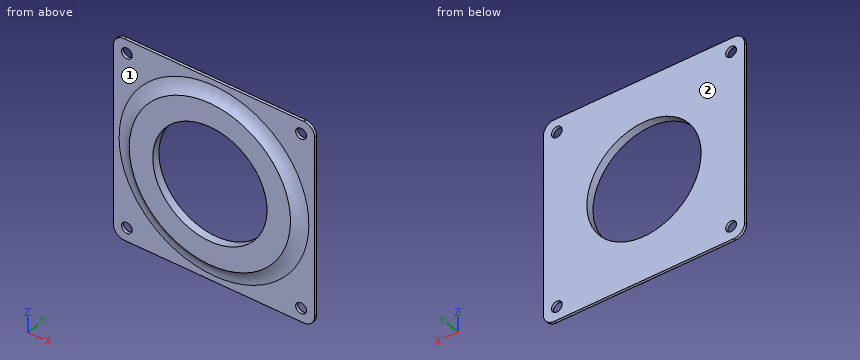
from build123d import *

# Parameters (mm, degrees)
BOSS_EXTRUDE1_DEPTH = 1.27
SKETCH2_R           = 38.1
BOSS_EXTRUDE2_DEPTH = 2.54
FILLET1_R           = 10.16
SKETCH3_R           = 27
CUT_EXTRUDE1_DEPTH  = 68.28310412
SKETCH4_R           = 2.54
CUT_EXTRUDE2_DEPTH  = 68.28310412


with BuildPart() as part:
    # Sketch1 → Boss-Extrude1 (new body)
    with BuildSketch(Plane(origin=(0, 0, 0), x_dir=(1, 0, 0), z_dir=(0, 1, 0))):
        with BuildLine():
            Line((-42.42, -47.5), (42.42, -47.5))
            ThreePointArc((42.42, -47.5), (46.012102448, -46.012102448), (47.5, -42.42))
            Line((47.5, -42.42), (47.5, 42.42))
            ThreePointArc((47.5, 42.42), (46.012102448, 46.012102448), (42.42, 47.5))
            Line((42.42, 47.5), (-42.42, 47.5))
            ThreePointArc((-42.42, 47.5), (-46.012102448, 46.012102448), (-47.5, 42.42))
            Line((-47.5, 42.42), (-47.5, -42.42))
            ThreePointArc((-47.5, -42.42), (-46.012102448, -46.012102448), (-42.42, -47.5))
        make_face()
    extrude(amount=BOSS_EXTRUDE1_DEPTH)

    # Sketch2 → Boss-Extrude2 (add)
    with BuildSketch(Plane.XZ):
        with Locations(Location((0, 0, 0), (0, 0, 270))):
            Circle(SKETCH2_R)
    extrude(amount=BOSS_EXTRUDE2_DEPTH)

    # Fillet1
    # the kernel refuses this fillet: 10.16 mm, written as the material it adds along each edge
    with BuildSketch(Plane(origin=(0, 0, 0), x_dir=(0, 0, -1), z_dir=(-1, 0, 0))) as fillet1_piece_1:
        with BuildLine():
            CenterArc((44.82020833, 10.16), FILLET1_R, 228.590377891, 41.409622109)
            Line((38.1, 2.54), (38.1, 0))
            Line((38.1, 0), (44.82020833, 0))
        make_face()
    revolve(axis=Axis((0, 0, 0), (0, -1, 0)))

    # Sketch3 → Cut-Extrude1 (cut, through all)
    with BuildSketch(Plane(origin=(0, 1.27, 0), x_dir=(1, 0, 0), z_dir=(0, 1, 0))):
        with Locations(Location((0, 0, 0), (0, 0, 270))):
            Circle(SKETCH3_R)
    extrude(amount=-CUT_EXTRUDE1_DEPTH, mode=Mode.SUBTRACT)

    # Sketch4 → Cut-Extrude2 (cut, through all)
    with BuildSketch(Plane(origin=(0, 1.27, 0), x_dir=(1, 0, 0), z_dir=(0, 1, 0))):
        with Locations(Location((-41.15, 41.15, 0), (0, 0, 270))):
            Circle(SKETCH4_R)
        with Locations(Location((41.15, 41.15, 0), (0, 0, 90))):
            Circle(SKETCH4_R)
        with Locations(Location((-41.15, -41.15, 0), (0, 0, 90))):
            Circle(SKETCH4_R)
        with Locations(Location((41.15, -41.15, 0), (0, 0, 270))):
            Circle(SKETCH4_R)
    extrude(amount=-CUT_EXTRUDE2_DEPTH, mode=Mode.SUBTRACT)


solid = part.part
Verification items for the finished model (mm, model axes). Face numbers are marked on the shaded views. A direction names the side the tool comes from. Coordinates: 2 decimals unless noted, no trailing zeros. Loops run counter-clockwise (first coordinate to the right, second up) from the corner with the lowest first, then second, coordinate; pieces in that order, holes last. Notation, with made-up numbers: (35.25, 27.25) -> (91.25, 27.25) arc R21 cw to (91.25, 63.25) -> close; hole circle Ø8 at (44.25, 31.5). An arc over 180 degrees is marked (long way). Answer as a JSON object with one key per item and string values. Group by question number.
Item 1: Sectioned sample at D-D on x = 41.15. State how many separate pieces and enclosed holes the cut face has, plus the area to 3 significant figures.
Item 2: Depth check by flat-ended pin: pin 1 (4.5 mm diameter, centred on x = -41.15, z = -41.15, fed in from +Y); pin 2 (6 mm diameter, centred on x = -41.15, z = 41.15, fed in from -Y). Enter the tip coordinate at first touch or a pass-through.
Item 3: Scan lines: probe 1 along X at (y, z) = (0.35, -41.15); probe 2 along X at (y, z) = (0.35, -1); probe 3 along X at (y, z) = (0.1, 23). Record each from-to range of solid material in increasing order.
Item 4: Sectioned sample at B-B on x = 0. Record the boundary of the cut face in (y, z), plus the area to 3 significant figures.
Item 5: Tool access check on the marked faces 1 and 2. Record the directions out of +Z, -Z, +X, -X, +Y, -Y that give a thin tool (end or side, any length) a straight path to the whole face; none if there is none.
Item 6: Sectioned sample at A-A on z = 0. Record the boundary of the cut face in (x, y).
Item 7: Sectioned sample at C-C on y = -0.6. Record the boundary of the cut face in (x, z).
Evaluation:
{
 "1": {"separate pieces": "3", "enclosed holes": "0", "area": "120 mm²"},
 "2": {"pin 1": "passes through", "pin 2": "stops at y = 0"},
 "3": {"probe 1": "x = -47.5 to -43.69, -38.61 to 38.61, 43.69 to 47.5", "probe 2": "x = -47.5 to -26.98, 26.98 to 47.5", "probe 3": "x = -47.5 to -14.14, 14.14 to 47.5"},
 "4": {"outline": "(-2.54, -38.1) arc R10.16 cw to (0, -44.82) -> (0, -47.5) -> (1.27, -47.5) -> (1.27, -27) -> (-2.54, -27) -> close; (-2.54, 27) -> (1.27, 27) -> (1.27, 47.5) -> (0, 47.5) -> (0, 44.82) arc R10.16 cw to (-2.54, 38.1) -> close", "area": "119 mm²"},
 "5": {"face 1": "-Y", "face 2": "+Z, -Z, +X, -X, +Y"},
 "6": {"outline": "(-47.5, 0) -> (-44.82, 0) arc R10.16 cw to (-38.1, -2.54) -> (-27, -2.54) -> (-27, 1.27) -> (-47.5, 1.27) -> close; (27, -2.54) -> (38.1, -2.54) arc R10.16 cw to (44.82, 0) -> (47.5, 0) -> (47.5, 1.27) -> (27, 1.27) -> close"},
 "7": {"outline": "circle Ø82.76 at (0, 0); hole circle Ø54 at (0, 0)"}
}
